Can you work these out from the model? Positions are in its coordinate system, mm. Face numbers are marked on the shaded views. A direction names the side the tool comes from. Round coordinates to 2 decimals unless told otherwise and drop trailing zeros. Loops run counter-clockwise (first coordinate to the right, second up) from the corner with the lowest first, then second, coordinate; pieces in that order, holes last.
(1) I want a section at D-D on x = 0.65. Write out the boundary of the cut face in (y, z), plus the area to 3 significant figures.
(2) If I drill on line 1 along X through (y, z) = (-1, 4); line 2 along Z through (x, y) = (3.7, 0.5); line 3 along Z through (x, y) = (0.35, 2.25), over which ranges is the centre line in solid material (lowest first)?
(3) I want a section at A-A on z = 0. Write out the boundary of the cut face in (x, y).
(4) Will these pins go through, and if not, where does the flat tip stop? pin 1 Ø1.5 at (x, z) = (5, 2.5) entering from +Y; pin 2 Ø3 at (x, z) = (1.5, 3) entering from +Y.
(5) I want a section at C-C on x = 4.3. Write out the boundary of the cut face in (y, z), plus the area to 3 significant figures.
(6) Which directions (+Z, -Z, +X, -X, +Y, -Y) give clear straight access to the entire face, cutting with the end or side of a thin tool? Please do the marked faces 1 and 2.
from build123d import *


with BuildPart() as part:
    # Sketch 1 → Revolve 1 (revolve)
    with BuildSketch(Plane.XY, mode=Mode.PRIVATE) as revolve_1_sk:
        with BuildLine():
            Line((0, 0), (0, 8))
            ThreePointArc((0, 8), (1.414213562, 7.414213562), (2, 6))
            Line((2, 6), (2, 3.5))
            ThreePointArc((2, 3.5), (2.146446609, 3.146446609), (2.5, 3))
            Line((2.5, 3), (5, 3))
            ThreePointArc((5, 3), (5.707106781, 2.707106781), (6, 2))
            Line((6, 2), (6, 0.7))
            ThreePointArc((6, 0.7), (5.505025253, 0.494974747), (5.3, 0))
            Line((5.3, 0), (0, 0))
        make_face()
    revolve(revolve_1_sk.sketch.rotate(Axis((6, 0, 0), (-1, 0, 0)), 180), axis=Axis((6, 0, 0), (-1, 0, 0)))


solid = part.part
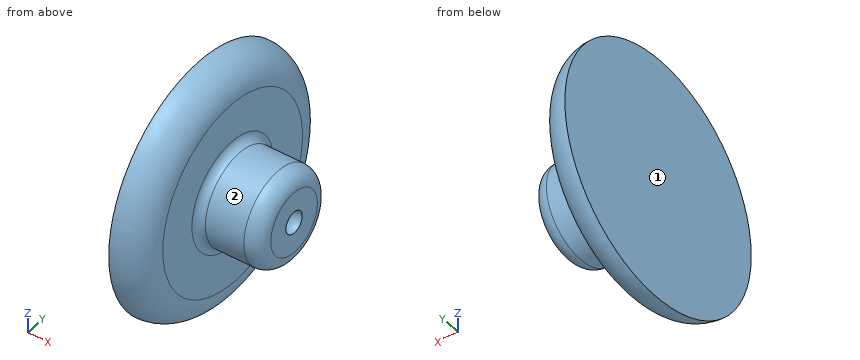
Filled sheet:
1. outline: circle Ø15.78 at (0, 0)
1. area: 196 mm2
2. line 1: x = 0 to 2
2. line 2: z = -2.96 to 2.96
2. line 3: z = -7.64 to 7.64
3. outline: (0, -8) arc R2 ccw to (2, -6) - (2, -3.5) arc R0.5 cw to (2.5, -3) - (5, -3) arc R1 ccw to (6, -2) - (6, -0.7) arc R0.7 cw to (6, 0.7) - (6, 2) arc R1 ccw to (5, 3) - (2.5, 3) arc R0.5 cw to (2, 3.5) - (2, 6) arc R2 ccw to (0, 8) - close
4. pin 1: stops at y = 2.44
4. pin 2: stops at y = 7.71
5. outline: circle Ø6 at (0, 0)
5. area: 28.3 mm2
6. face 1: +Z, -Z, -X, +Y, -Y
6. face 2: +X
